```python
from build123d import *
from build123d import SkipClean  # not in build123d's __all__

# Parameters (mm, degrees)
F2_R     = 20.3469556015
F2_R_2   = 13
F2_R_3   = 3
F3_DEPTH = 3


with BuildPart() as f1:
    # F0 (on Right) → F1 (revolve)
    with BuildSketch(Plane.YZ):
        with BuildLine():
            Line((-3, -5), (-3, 0))
            Line((-3, 0), (-3, 5))
            Line((-3, 5), (-13, 5))
            Line((-13, 5), (-13, 4))
            ThreePointArc((-13, 4), (-11, 0), (-13, -4))
            Line((-13, -4), (-13, -5))
            Line((-13, -5), (-3, -5))
        make_face()
    revolve(axis=Axis((0, 0, 3.2237173374), (0, 0, 1)))

    # F2 (on face) → F3 (join)
    with BuildSketch(Plane(origin=(0, 0, -5), x_dir=(1, 0, 0), z_dir=(0, 0, -1))):
        Circle(F2_R)
        Circle(F2_R_2, mode=Mode.SUBTRACT)
        Circle(F2_R_2)
        Circle(F2_R_3, mode=Mode.SUBTRACT)
    with SkipClean():  # cleaning this boolean's faces spoils the solid; the shape is the same uncleaned
        extrude(amount=F3_DEPTH)


solid = f1.part
```
Design review of the part built by this model. Coordinates are the model's own, in mm. A direction names the side the tool comes from. Coordinates: 2 decimals unless noted, no trailing zeros. Loops run counter-clockwise (first coordinate to the right, second up) from the corner with the lowest first, then second, coordinate; pieces in that order, holes last. Notation, with made-up numbers: (82.5, 79) - (97.5, 79) arc R15 cw to (97.5, 93) - close; hole circle Ø3 at (43.5, 82). An arc over 180 degrees is marked (long way). Use CSV: the item, a comma, the result in double quotes. Start each with the question number.
1) Tool access review of faces 1 (the cylindrical face through (-16.147, 12.381, -6.479)), 2 (the cylindrical face through (-7.91, 10.316, 4.493)): name each direction out of +Z, -Z, +X, -X, +Y, -Y from which nothing blocks a thin tool from reaching the whole face with its end or side.
2) Consider section D-D on z = 1. Write out the cut boundary in (x, y), then the cut area to 3 significant figures.
3) Consider section B-B on y = -14. Write out the cut boundary in (x, z).
4) For pin 1 Ø6 at (y, z) = (-9.5, -6) entering from +X; pin 2 Ø5 at (x, y) = (-10.5, -16) entering from +Z, all flat-tipped, find the tip position at first contact; note any pin that passes through.
5) Wall thickness on L1, parallel to Y at x = 0, z = -5.75; L2, parallel to Z at x = -11.5, y = -4.5; L3, parallel to X at y = 0, z = -0.25: over which ranges is each line inside the solid? List them lowest first. Write a range as from..to.
Geometry says:
1,face 1,"+Z, -Z"
1,face 2,"+Z"
2,outline,"circle Ø22.2 at (0, 0); hole circle Ø6 at (0, 0)"
2,area,"359 mm^2"
3,outline,"(-14.76, -8) - (14.76, -8) - (14.76, -5) - (-14.76, -5) - close"
4,pin 1,"x = 19.28"
4,pin 2,"z = -5"
5,L1,"-20.35..-3, 3..20.35"
5,L2,"-8..-3.42, 3.42..5"
5,L3,"-11.01..-3, 3..11.01"
